```python
from build123d import *

# Parameters (mm, degrees)
F0_R     = 11.1125
F1_DEPTH = 6.35
F2_R     = 3.17499
F3_DEPTH = 7


# Not quite as in the source:
# - a fillet or chamfer is up to 0.001 mm smaller than in the source, because OpenCascade refuses the exact size


with BuildPart() as f1:
    # F0 (on Top) → F1 (new body)
    with BuildSketch(Plane.XY):
        with BuildLine():
            ThreePointArc((-9.9264482926, -9.8298791597), (-7.1913775024, -11.9768522417), (-4.010805007, -13.3818662075))
            ThreePointArc((-4.010805007, -13.3818662075), (-3.9641218469, -13.3957694062), (-3.9173904939, -13.4095097494))
            ThreePointArc((-3.9173904939, -13.4095097494), (0, -13.97), (3.9173904939, -13.4095097494))
            ThreePointArc((3.9173904939, -13.4095097494), (7.1495738947, -12.001853737), (9.9264482926, -9.8298791597))
            ThreePointArc((9.9264482926, -9.8298791597), (12.4120380065, -6.4111007266), (13.7613551332, -2.4054115859))
            ThreePointArc((13.7613551332, -2.4054115859), (13.5892538356, -1.2081742794), (13.5317131076, 0))
            Line((13.5317131076, 0), (11.1125, 0))
            ThreePointArc((11.1125, 0), (0, -11.1125), (-11.1125, 0))
            Line((-11.1125, 0), (-13.5317149703, 0))
            ThreePointArc((-13.5317149703, 0), (-13.589255453, -1.2081717101), (-13.7613560192, -2.4054065173))
            ThreePointArc((-13.7613560192, -2.4054065173), (-12.4120391871, -6.4110984408), (-9.9264482926, -9.8298791597))
        make_face()
        with BuildLine():
            ThreePointArc((3.9173904939, -13.4095097494), (0, -13.97), (-3.9173904939, -13.4095097494))
            Line((-3.9173904939, -13.4095097494), (0, -21.4545894414))
            Line((0, -21.4545894414), (3.9173904939, -13.4095097494))
        make_face()
        with BuildLine():
            ThreePointArc((-12.6513041413, -21.8456521056), (-14.7063688094, -15.0627697401), (-9.9264482926, -9.8298791597))
            ThreePointArc((-9.9264482926, -9.8298791597), (-12.4120391871, -6.4110984408), (-13.7613560192, -2.4054065173))
            ThreePointArc((-13.7613560192, -2.4054065173), (-13.9177412605, -1.2072192038), (-13.97, 0))
            ThreePointArc((-13.97, 0), (-13.9177412605, 1.2072192038), (-13.7613560192, 2.4054065173))
            ThreePointArc((-13.7613560192, 2.4054065173), (-12.4120395648, 6.4110977096), (-9.9264494507, 9.8298779902))
            ThreePointArc((-9.9264494507, 9.8298779902), (-18.1475057056, 13.8110021796), (-18.2071019663, 22.9450902043))
            ThreePointArc((-18.2071019663, 22.9450902043), (-30.3564318276, 19.9035068059), (-40.5314124536, 12.6009582845))
            ThreePointArc((-40.5314124536, 12.6009582845), (-45.1838875342, -2.0490994228), (-37.5057111895, -15.3650794177))
            ThreePointArc((-37.5057111895, -15.3650794177), (-25.7855371398, -21.3169777129), (-12.6513041413, -21.8456521056))
        make_face()
        with Locations((-26.2444149703, 0)):
            Circle(F0_R, mode=Mode.SUBTRACT)
        with BuildLine():
            ThreePointArc((13.7613551332, -2.4054115859), (12.4120380065, -6.4111007266), (9.9264482926, -9.8298791597))
            ThreePointArc((9.9264482926, -9.8298791597), (14.7063688094, -15.0627697401), (12.6513041413, -21.8456521056))
            ThreePointArc((12.6513041413, -21.8456521056), (25.7855371398, -21.3169777129), (37.5057111895, -15.3650794177))
            ThreePointArc((37.5057111895, -15.3650794177), (43.2360320484, -8.6132099574), (45.2944131076, 0))
            Line((45.2944131076, 0), (37.3569131076, 0))
            ThreePointArc((37.3569131076, 0), (26.2444131076, -11.1125), (15.1319131076, 0))
            Line((15.1319131076, 0), (13.97, 0))
            ThreePointArc((13.97, 0), (13.9177410382, -1.2072217669), (13.7613551332, -2.4054115859))
        make_face()
        with BuildLine():
            ThreePointArc((-13.7613560192, 2.4054065173), (-13.589255453, 1.2081717101), (-13.5317149703, 0))
            Line((-13.5317149703, 0), (-11.1125, 0))
            ThreePointArc((-11.1125, 0), (0, 11.1125), (11.1125, 0))
            Line((11.1125, 0), (13.5317131076, 0))
            ThreePointArc((13.5317131076, 0), (13.5892538356, 1.2081742794), (13.7613551332, 2.4054115859))
            ThreePointArc((13.7613551332, 2.4054115859), (12.4120383841, 6.4110999954), (9.9264494507, 9.8298779902))
            ThreePointArc((9.9264494507, 9.8298779902), (7.1495746018, 12.0018533158), (3.9173904939, 13.4095097494))
            ThreePointArc((3.9173904939, 13.4095097494), (2.4938325804, 13.7456065367), (1.0429356844, 13.9310152235))
            ThreePointArc((1.0429356844, 13.9310152235), (0, 13.97), (-1.0429356844, 13.9310152235))
            ThreePointArc((-1.0429356844, 13.9310152235), (-2.4938325804, 13.7456065367), (-3.9173904939, 13.4095097494))
            ThreePointArc((-3.9173904939, 13.4095097494), (-7.1495746018, 12.0018533158), (-9.9264494507, 9.8298779902))
            ThreePointArc((-9.9264494507, 9.8298779902), (-12.4120395648, 6.4110977096), (-13.7613560192, 2.4054065173))
        make_face()
        with BuildLine():
            ThreePointArc((13.7613551332, 2.4054115859), (13.9177410382, 1.2072217669), (13.97, 0))
            Line((13.97, 0), (15.1319131076, 0))
            ThreePointArc((15.1319131076, 0), (26.2444131076, 11.1125), (37.3569131076, 0))
            Line((37.3569131076, 0), (45.2944131076, 0))
            ThreePointArc((45.2944131076, 0), (44.0639226062, 6.7355460973), (40.5314124536, 12.6009582845))
            ThreePointArc((40.5314124536, 12.6009582845), (30.3564318276, 19.9035068059), (18.2071019663, 22.9450902043))
            ThreePointArc((18.2071019663, 22.9450902043), (18.1475057056, 13.8110021796), (9.9264494507, 9.8298779902))
            ThreePointArc((9.9264494507, 9.8298779902), (12.4120383841, 6.4110999954), (13.7613551332, 2.4054115859))
        make_face()
        with BuildLine():
            Line((-3.102583345, 18.8314262778), (-3.9173904939, 13.4095097494))
            ThreePointArc((-3.9173904939, 13.4095097494), (-2.4938325804, 13.7456065367), (-1.0429356844, 13.9310152235))
            Line((-1.0429356844, 13.9310152235), (-3.102583345, 18.8314262778))
        make_face()
        with BuildLine():
            ThreePointArc((1.0429356844, 13.9310152235), (2.4938325804, 13.7456065367), (3.9173904939, 13.4095097494))
            Line((3.9173904939, 13.4095097494), (3.102583345, 18.8314262778))
            Line((3.102583345, 18.8314262778), (1.0429356844, 13.9310152235))
        make_face()
    extrude(amount=F1_DEPTH)

    # F2 (radius 3.175 in the source; OpenCascade refuses exactly that, so slightly less here)
    f2_edges = [f1.edges().sort_by_distance(p)[0] for p in [
        (-45.183888, -2.049099, 6.35),
        (45.183888, -2.049099, 6.35),
        (45.183888, -2.049099, 0),
        (-45.183888, -2.049099, 0),
    ]]
    fillet(f2_edges, radius=F2_R)

    # F0 (on Top) → F3 (join)
    with BuildSketch(Plane.XY):
        with BuildLine():
            ThreePointArc((-9.9264482926, -9.8298791597), (-7.1913775024, -11.9768522417), (-4.010805007, -13.3818662075))
            ThreePointArc((-4.010805007, -13.3818662075), (-3.9641218469, -13.3957694062), (-3.9173904939, -13.4095097494))
            ThreePointArc((-3.9173904939, -13.4095097494), (0, -13.97), (3.9173904939, -13.4095097494))
            ThreePointArc((3.9173904939, -13.4095097494), (7.1495738947, -12.001853737), (9.9264482926, -9.8298791597))
            ThreePointArc((9.9264482926, -9.8298791597), (12.4120380065, -6.4111007266), (13.7613551332, -2.4054115859))
            ThreePointArc((13.7613551332, -2.4054115859), (13.5892538356, -1.2081742794), (13.5317131076, 0))
            Line((13.5317131076, 0), (11.1125, 0))
            ThreePointArc((11.1125, 0), (0, -11.1125), (-11.1125, 0))
            Line((-11.1125, 0), (-13.5317149703, 0))
            ThreePointArc((-13.5317149703, 0), (-13.589255453, -1.2081717101), (-13.7613560192, -2.4054065173))
            ThreePointArc((-13.7613560192, -2.4054065173), (-12.4120391871, -6.4110984408), (-9.9264482926, -9.8298791597))
        make_face()
        with BuildLine():
            ThreePointArc((3.9173904939, -13.4095097494), (0, -13.97), (-3.9173904939, -13.4095097494))
            Line((-3.9173904939, -13.4095097494), (0, -21.4545894414))
            Line((0, -21.4545894414), (3.9173904939, -13.4095097494))
        make_face()
        with BuildLine():
            ThreePointArc((-12.6513041413, -21.8456521056), (-14.7063688094, -15.0627697401), (-9.9264482926, -9.8298791597))
            ThreePointArc((-9.9264482926, -9.8298791597), (-12.4120391871, -6.4110984408), (-13.7613560192, -2.4054065173))
            ThreePointArc((-13.7613560192, -2.4054065173), (-13.9177412605, -1.2072192038), (-13.97, 0))
            ThreePointArc((-13.97, 0), (-13.9177412605, 1.2072192038), (-13.7613560192, 2.4054065173))
            ThreePointArc((-13.7613560192, 2.4054065173), (-12.4120395648, 6.4110977096), (-9.9264494507, 9.8298779902))
            ThreePointArc((-9.9264494507, 9.8298779902), (-18.1475057056, 13.8110021796), (-18.2071019663, 22.9450902043))
            ThreePointArc((-18.2071019663, 22.9450902043), (-30.3564318276, 19.9035068059), (-40.5314124536, 12.6009582845))
            ThreePointArc((-40.5314124536, 12.6009582845), (-45.1838875342, -2.0490994228), (-37.5057111895, -15.3650794177))
            ThreePointArc((-37.5057111895, -15.3650794177), (-25.7855371398, -21.3169777129), (-12.6513041413, -21.8456521056))
        make_face()
        with Locations((-26.2444149703, 0)):
            Circle(F0_R, mode=Mode.SUBTRACT)
        with BuildLine():
            ThreePointArc((13.7613551332, -2.4054115859), (12.4120380065, -6.4111007266), (9.9264482926, -9.8298791597))
            ThreePointArc((9.9264482926, -9.8298791597), (14.7063688094, -15.0627697401), (12.6513041413, -21.8456521056))
            ThreePointArc((12.6513041413, -21.8456521056), (25.7855371398, -21.3169777129), (37.5057111895, -15.3650794177))
            ThreePointArc((37.5057111895, -15.3650794177), (43.2360320484, -8.6132099574), (45.2944131076, 0))
            Line((45.2944131076, 0), (37.3569131076, 0))
            ThreePointArc((37.3569131076, 0), (26.2444131076, -11.1125), (15.1319131076, 0))
            Line((15.1319131076, 0), (13.97, 0))
            ThreePointArc((13.97, 0), (13.9177410382, -1.2072217669), (13.7613551332, -2.4054115859))
        make_face()
        with BuildLine():
            ThreePointArc((-13.7613560192, 2.4054065173), (-13.589255453, 1.2081717101), (-13.5317149703, 0))
            Line((-13.5317149703, 0), (-11.1125, 0))
            ThreePointArc((-11.1125, 0), (0, 11.1125), (11.1125, 0))
            Line((11.1125, 0), (13.5317131076, 0))
            ThreePointArc((13.5317131076, 0), (13.5892538356, 1.2081742794), (13.7613551332, 2.4054115859))
            ThreePointArc((13.7613551332, 2.4054115859), (12.4120383841, 6.4110999954), (9.9264494507, 9.8298779902))
            ThreePointArc((9.9264494507, 9.8298779902), (7.1495746018, 12.0018533158), (3.9173904939, 13.4095097494))
            ThreePointArc((3.9173904939, 13.4095097494), (2.4938325804, 13.7456065367), (1.0429356844, 13.9310152235))
            ThreePointArc((1.0429356844, 13.9310152235), (0, 13.97), (-1.0429356844, 13.9310152235))
            ThreePointArc((-1.0429356844, 13.9310152235), (-2.4938325804, 13.7456065367), (-3.9173904939, 13.4095097494))
            ThreePointArc((-3.9173904939, 13.4095097494), (-7.1495746018, 12.0018533158), (-9.9264494507, 9.8298779902))
            ThreePointArc((-9.9264494507, 9.8298779902), (-12.4120395648, 6.4110977096), (-13.7613560192, 2.4054065173))
        make_face()
        with BuildLine():
            ThreePointArc((13.7613551332, 2.4054115859), (13.9177410382, 1.2072217669), (13.97, 0))
            Line((13.97, 0), (15.1319131076, 0))
            ThreePointArc((15.1319131076, 0), (26.2444131076, 11.1125), (37.3569131076, 0))
            Line((37.3569131076, 0), (45.2944131076, 0))
            ThreePointArc((45.2944131076, 0), (44.0639226062, 6.7355460973), (40.5314124536, 12.6009582845))
            ThreePointArc((40.5314124536, 12.6009582845), (30.3564318276, 19.9035068059), (18.2071019663, 22.9450902043))
            ThreePointArc((18.2071019663, 22.9450902043), (18.1475057056, 13.8110021796), (9.9264494507, 9.8298779902))
            ThreePointArc((9.9264494507, 9.8298779902), (12.4120383841, 6.4110999954), (13.7613551332, 2.4054115859))
        make_face()
        with BuildLine():
            Line((-3.102583345, 18.8314262778), (-3.9173904939, 13.4095097494))
            ThreePointArc((-3.9173904939, 13.4095097494), (-2.4938325804, 13.7456065367), (-1.0429356844, 13.9310152235))
            Line((-1.0429356844, 13.9310152235), (-3.102583345, 18.8314262778))
        make_face()
        with BuildLine():
            ThreePointArc((1.0429356844, 13.9310152235), (2.4938325804, 13.7456065367), (3.9173904939, 13.4095097494))
            Line((3.9173904939, 13.4095097494), (3.102583345, 18.8314262778))
            Line((3.102583345, 18.8314262778), (1.0429356844, 13.9310152235))
        make_face()
    extrude(amount=F3_DEPTH)


solid = f1.part
```
The listing builds one solid part. Answer for the finished solid, in the listing's coordinates (mm). A direction names the side the tool comes from. Round coordinates to 2 decimals unless told otherwise and drop trailing zeros. Order: outer loops, then holes, each group sorted by start corner. A loop starts at its lowest first (then second) coordinate and runs counter-clockwise, first axis right, second up. Notation, with made-up numbers: (35, 14) - (51, 14) arc R23 ccw to (51, 49) - close; hole circle Ø1 at (80.5, -7.75). An arc over 180 degrees is marked (long way). Put each result on its own line as item: value. Start each with the question number.
(1) Find section C-C (y = -9). Give the vertices of the cut face in (x, z), plus the area to 3 significant figures.
(2) Straight lines are drawn through the part: probe 1 along X at (y, z) = (1.5, 3.25); probe 2 along X at (y, z) = (7, 5); probe 3 along X at (y, z) = (-2.5, 2). For each, find the intervals that lie inside material, in ascending order. Write a range as from..to.
(3) Find section B-B (x = -16). Give the vertices of the cut face in (y, z), plus the area to 3 significant figures.
(4) Given P1, Ø1.5, axis at y = -3.5, z = 6, coming from the -X side; P2, Ø3, axis at y = 6, z = 6, coming from the +X side, each flat-ended and moving along its own axis, determine where each tip first touches the part or whether it passes through.
(5) Find section D-D (x = -32). Give the vertices of the cut face in (y, z), plus the area to 3 significant figures.
(6) Find section A-A (z = 2). State how many separate pieces and enclosed holes the cut face has, plus the area to 3 significant figures.
(7) For faces 1 (the cylindrical face through (37.346, 0.489, 3.451)), 2 (the flat face through (1.93, -17.49, 3.45)), 3 (the flat face through (2.09, 16.42, 3.45)), determine the directions among +Z, -Z, +X, -X, +Y, -Y from which every point of the face is accessible in a straight line to the end or side of a thin tool.
Reply:
1. outline: (-43.03, 0) - (-32.76, 0) - (-32.76, 7) - (-43.03, 7) - close; (-19.73, 0) - (-6.52, 0) - (-6.52, 7) - (-19.73, 7) - close; (6.52, 0) - (19.73, 0) - (19.73, 7) - (6.52, 7) - close; (32.76, 0) - (43.03, 0) - (43.03, 7) - (32.76, 7) - close
1. area: 329 mm^2
2. probe 1: -45.24..-37.26, -15.23..-13.89, -13.62..-11.01, 11.01..13.62, 13.89..15.23, 37.26..45.24
2. probe 2: -43.96..-34.88, -17.61..-8.63, 8.63..17.61, 34.88..43.96
2. probe 3: -45.13..-37.07, -15.42..-10.83, 10.83..15.42, 37.07..45.13
3. outline: (-22.25, 0) - (-4.31, 0) - (-4.31, 7) - (-22.25, 7) - close; (4.31, 0) - (11.49, 0) - (11.49, 7) - (4.31, 7) - close
3. area: 176 mm^2
4. P1: x = -45.09
4. P2: x = 44.76
5. outline: (-18.96, 0) - (-9.51, 0) - (-9.51, 7) - (-18.96, 7) - close; (9.51, 0) - (19.09, 0) - (19.09, 7) - (9.51, 7) - close
5. area: 133 mm^2
6. separate pieces: 1
6. enclosed holes: 5
6. area: 1,710 mm^2
7. face 1: +Z, -Z
7. face 2: +Z, -Z, -Y
7. face 3: +Z, -Z, +Y
